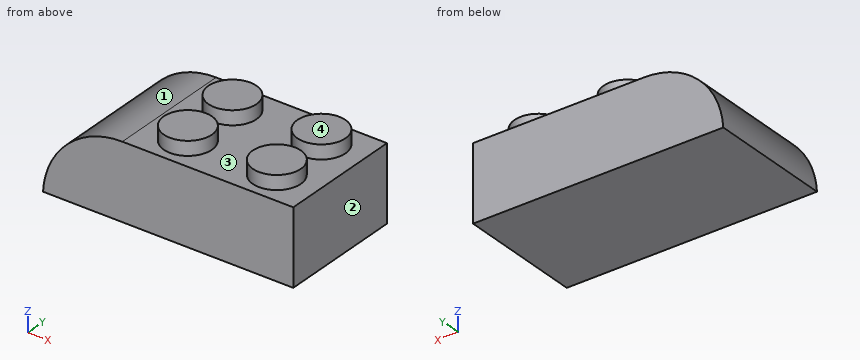
from build123d import *

# Parameters (mm, degrees)
F0_W        = 32
F0_H        = 16
F1_DEPTH    = 9.6
F2_T1_DEPTH = 66.7227759493
F3_R        = 3.0688775333
F4_DEPTH    = 1.8


# Not quite as in the source:
# - a fillet or chamfer that OpenCascade refuses, or shapes differently, is made with other operations: its cross-section is extruded or revolved along the edge and cut away or added
# - a feature names something its author has since deleted; it is built from what else it names


with BuildPart() as f1:
    # F0 (on Top) → F1 (new body)
    with BuildSketch(Plane.XY):
        with Locations((-16, 8)):
            Rectangle(F0_W, F0_H)
    extrude(amount=F1_DEPTH)

    # F2: fillet of radius 10.16 on 1 edges, made by hand

    # F2_s2 → F2_t1 (cut)
    with BuildSketch(Plane.XZ.offset(-41.3613879746)):
        with BuildLine():
            ThreePointArc((-32, 0), (-28.8388537198, 6.819539281), (-21.8554448101, 9.6))
            Line((-21.8554448101, 9.6), (-32, 9.6))
            Line((-32, 9.6), (-32, 0))
        make_face()
    extrude(amount=F2_T1_DEPTH, mode=Mode.SUBTRACT)

    # F3 (on face) → F4 (join)
    with BuildSketch(Plane.XY.offset(9.6)):
        with Locations((-16.6150905888, 11.8076978251)):
            Circle(F3_R)
        with Locations((-5.2403542213, 11.8076978251)):
            Circle(F3_R)
        with Locations((-16.6150905888, 4.1923021749)):
            Circle(F3_R)
        with Locations((-5.2403542213, 4.1923021749)):
            Circle(F3_R)
    extrude(amount=F4_DEPTH)


solid = f1.part
The model under review builds one solid part; all positions refer to its coordinate system, in mm. Face numbers are marked on the shaded views. Coordinates: 2 decimals unless noted, no trailing zeros. Write each loop counter-clockwise with the first axis right and the second up, starting at its lowest first coordinate (ties: lowest second). Pieces come first, ordered by that corner, then holes. Notation, with made-up numbers: M 82.5,63.25 L 92.5,63.25 A11 ccw 92.5,71.25 Z; hole C 21.5,55 d5. An arc over 180 degrees is marked long. Put each result on its own line as item: value.
1) Wall thickness on probe 1 along Z at (x, y) = (-1.5, 9.5); probe 2 along X at (y, z) = (1.75, 10.5); probe 3 along X at (y, z) = (5, 10.25): over which ranges is each line inside the solid? List them lowest first. Write a range as [from, to].
Computed:
probe 1: z = [0, 9.6]
probe 2: x = [-18.47, -14.76], [-7.1, -3.38]
probe 3: x = [-19.58, -13.65], [-8.2, -2.28]
2) Draft analysis for pull direction X (two halves, no side actions). For the marked faces 1, 2, 3 and 4, state which applies: released by +X, released by -X, zero draft, split by the parting line, or undercut.
Computed:
face 1: released by -X
face 2: released by +X
face 3: undercut
face 4: zero draft
3) Add section C-C on z = 5.75. Give the boundary of the cut face in (x, y), then the cut area to 3 significant figures.
Computed:
outline: M -29.82,0 L 0,0 L 0,16 L -29.82,16 Z
area: 477 mm2
4) Add section B-B on x = -18.5. Give the boundary of the cut face in (y, z).
Computed:
outline: M 0,0 L 16,0 L 16,9.6 L 14.23,9.6 L 14.23,11.4 L 9.39,11.4 L 9.39,9.6 L 6.61,9.6 L 6.61,11.4 L 1.77,11.4 L 1.77,9.6 L 0,9.6 Z
5) Add section A-A on y = 2. Give the boundary of the cut face in (x, z), then the cut area to 3 significant figures.
Computed:
outline: M -32,0 L 0,0 L 0,9.6 L -3.09,9.6 L -3.09,11.4 L -7.39,11.4 L -7.39,9.6 L -14.47,9.6 L -14.47,11.4 L -18.76,11.4 L -18.76,9.6 L -21.86,9.6 A10.16 ccw Z
area: 301 mm2
6) Clearance check with flat-ended pins moving along their axes: pin 1 Ø1.5 at (x, y) = (-14.5, 9.5) entering from -Z; pin 2 Ø5 at (y, z) = (8, 4) entering from -X; pin 3 Ø1.5 at (x, y) = (-6.5, 8) entering from +Z; pin 4 Ø1.5 at (y, z) = (6, 9.5) entering from -X. State where each tip first meets the part, or that it passes through.
Computed:
pin 1: stops at z = 0
pin 2: stops at x = -31.8
pin 3: stops at z = 9.6
pin 4: stops at x = -25.92
7) Add section D-D on x = -11.5. Give the boundary of the cut face in (y, z), then the cut area to 3 significant figures.
Computed:
outline: M 0,0 L 16,0 L 16,9.6 L 0,9.6 Z
area: 154 mm2
